Geometry: see drawing. Coordinates: mm, zero at the bounding-box minimum. Coordinates: 2 decimals unless noted, no trailing zeros. Order: outer loops, then holes, each group sorted by start corner. A loop starts at its lowest first (then second) coordinate and runs counter-clockwise, first axis right, second up.
Item 1: Mould query, pull axis Y, two halves, no side actions, for the marked faces 1, 2 and 3. Classes: released by +Y, released by -Y, zero draft, split by the parting line, or undercut.
Item 2: Section A-A on y = 2.54. Return the cut outline in (x, z) (3 decimals), then the cut area to 3 significant figures.
Item 3: Contact query for a flat-ended pin moving along its axis: P1, Ø1, axis at x = 1, y = 2.5, coming from the -Z side. Output: stop coordinate, or through.
Item 4: Ray query, line 1 (Y direction, x = 2.54, z = 6.5); line 2 (Z direction, x = 3.1, y = 1.3); line 3 (Z direction, x = 2.4, y = 2.7). Return the intervals inside material, ascending.
Item 5: Section C-C on z = 6.75. Return the cut outline in (x, y).
Item 6: Section D-D on x = 3.2. Return the cut outline in (y, z), then the cut area to 3 significant figures.
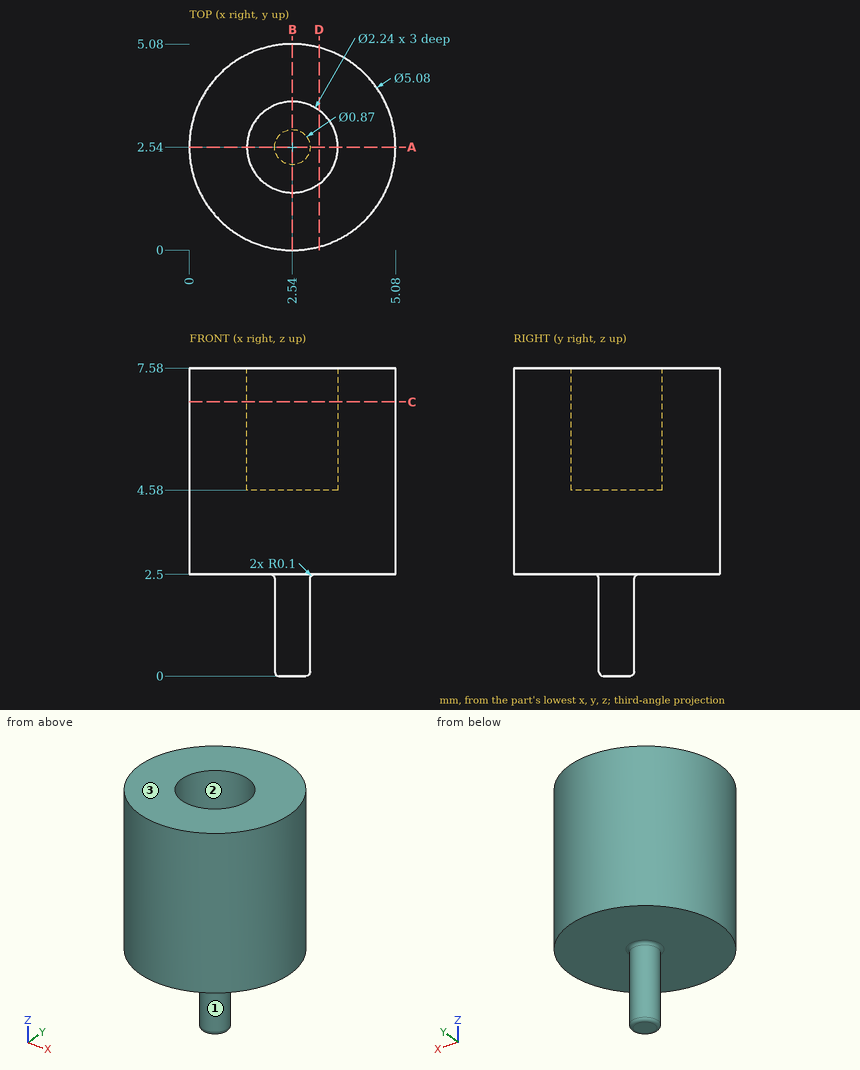
Answer list:
1. face 1: split by the parting line
1. face 2: undercut
1. face 3: zero draft
2. outline: (0, 2.5) - (2.005, 2.5) arc R0.1 cw to (2.105, 2.4) - (2.105, 0.1) arc R0.1 ccw to (2.205, 0) - (2.875, 0) arc R0.1 ccw to (2.975, 0.1) - (2.975, 2.4) arc R0.1 cw to (3.075, 2.5) - (5.08, 2.5) - (5.08, 7.58) - (3.66, 7.58) - (3.66, 4.58) - (1.42, 4.58) - (1.42, 7.58) - (0, 7.58) - close
2. area: 21.3 mm2
3. P1: stops at z = 2.5
4. line 1: y = 0 to 1.42, 3.66 to 5.08
4. line 2: z = 2.5 to 7.58
4. line 3: z = 0 to 4.58
5. outline: circle Ø5.08 at (2.54, 2.54); hole circle Ø2.24 at (2.54, 2.54)
6. outline: (0.09, 2.5) - (4.99, 2.5) - (4.99, 7.58) - (3.44, 7.58) - (3.44, 4.58) - (1.64, 4.58) - (1.64, 7.58) - (0.09, 7.58) - close
6. area: 19.5 mm2
